from build123d import *


with BuildPart() as f1:
    # F0 (on Front) → F1 (revolve)
    with BuildSketch(Plane.XZ):
        with BuildLine():
            Line((-19.05, 0), (0, 0))
            Line((0, 0), (0, 6.35))
            Line((0, 6.35), (-9.638313, 6.35))
            ThreePointArc((-9.638313, 6.35), (-10.007201, 6.502799), (-10.16, 6.871687))
            Line((-10.16, 6.871687), (-10.16, 7.67267))
            ThreePointArc((-10.16, 7.67267), (-10.452527, 8.293544), (-11.117546, 8.463267))
            ThreePointArc((-11.117546, 8.463267), (-14.691922, 7.657891), (-18.209131, 6.631224))
            ThreePointArc((-18.209131, 6.631224), (-18.426498, 6.520989), (-18.600173, 6.35))
            ThreePointArc((-18.600173, 6.35), (-18.749447, 5.984448), (-18.704121, 5.592202))
            ThreePointArc((-18.704121, 5.592202), (-18.269118, 2.7585), (-19.05, 0))
        make_face()
    revolve(axis=Axis((0, 0, 3.175), (0, 0, 1)))


solid = f1.part
Work out the finished part from the listing and answer in its coordinate system (mm). Round coordinates to 2 decimals unless told otherwise and drop trailing zeros. Order: outer loops, then holes, each group sorted by start corner. A loop starts at its lowest first (then second) coordinate and runs counter-clockwise, first axis right, second up. Notation, with made-up numbers: M 31,12 L 79,12 A19 ccw 79,23 Z; hole C 62.5,74.5 d2. An arc over 180 degrees is marked long. Put each result on its own line as item: value. Start each with the question number.
Q1. Flat-ended cylindrical pins translate along their axes: pin 1 (5 mm diameter, centred on y = 4, z = 6.5, fed in from -X); pin 2 (4 mm diameter, centred on x = -12.5, y = 5, fed in from +Z); pin 3 (1 mm diameter, centred on y = 11.5, z = 2, fed in from -X); pin 4 (21 mm diameter, centred on x = 3, y = -2, fed in from +Z). Find the tip coordinate at first contact, or state that the pin passes through.
Q2. Straight lines are drawn through the part: L1, parallel to Z at x = 8, y = -15.5; L2, parallel to Z at x = -5, y = -6; L3, parallel to Y at x = -8, z = 2.25. For each, find the intervals that lie inside material, in ascending order. Write a range as [from, to].
Q3. For a pull along Y with two mould halves and no side action, classify faces 1 (the flat face through (0, 0, 0)), 2 (the flat face through (0, 0, 6.35)) as pulls with the +Y half, pulls with the -Y half, needs draft (parallel to the pull), parting line crosses it, or undercut.
Q4. Section A-A, the plane z = 3.75 is taken. Write down the section's boundary in (x, y).
Q5. Section B-B, the plane z = 1 is taken. Write down the section's boundary in (x, y), and give its area (3 significant figures).
Findings below:
1. pin 1: stops at x = -18.69
1. pin 2: stops at z = 8.4
1. pin 3: stops at x = -14.72
1. pin 4: stops at z = 8.48
2. L1: z = [0, 6.88]
2. L2: z = [0, 6.35]
2. L3: y = [-16.48, 16.48]
3. face 1: needs draft
3. face 2: undercut
4. outline: C 0,0 d36.56
5. outline: C 0,0 d37.23
5. area: 1,090 mm^2
